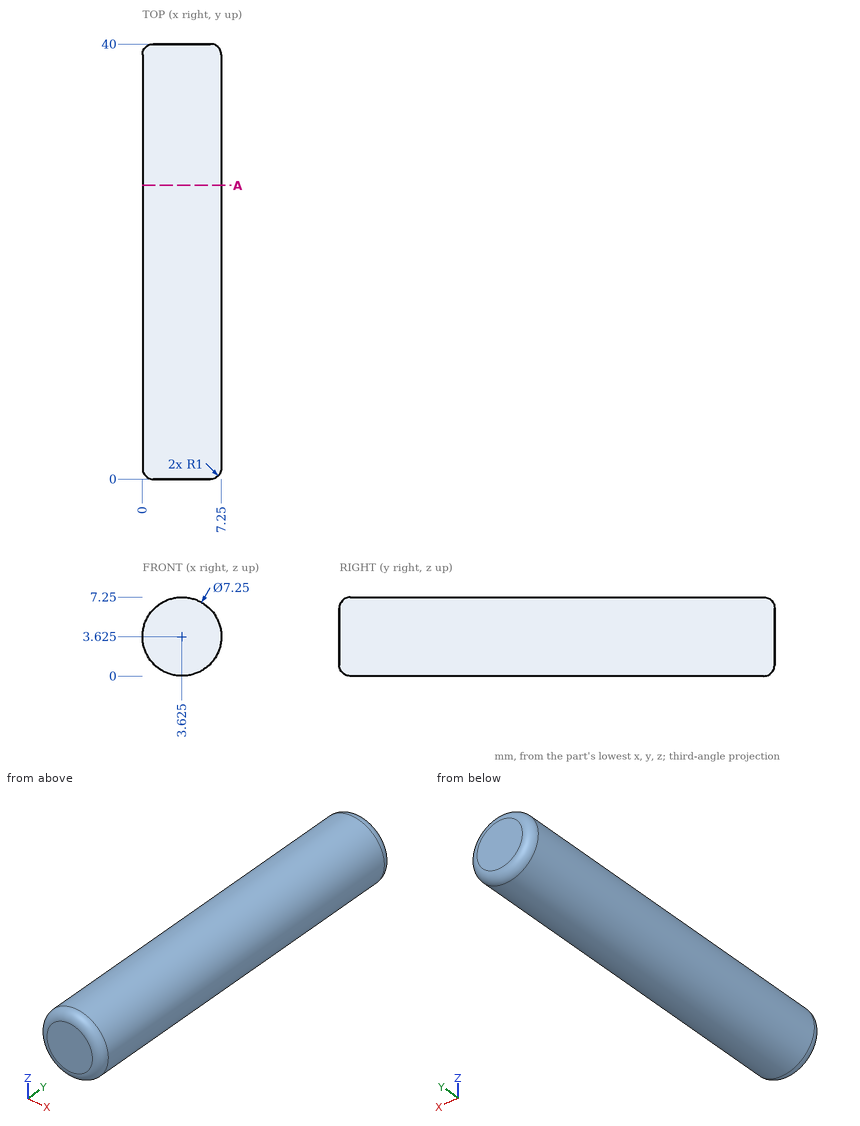
Design review of the part shown in the three views and the two pictorial views. Dimensions are in mm from the part's minimum x, y and z. Round coordinates to 2 decimals unless told otherwise and drop trailing zeros. Order: outer loops, then holes, each group sorted by start corner. A loop starts at its lowest first (then second) coordinate and runs counter-clockwise, first axis right, second up. Notation, with made-up numbers: (42.25, 7.25) - (57.25, 7.25) arc R22 cw to (57.25, 24.25) - close; hole circle Ø10 at (88.5, -19). An arc over 180 degrees is marked (long way). Answer in a Markdown table with one row per item.
(1) Clearance check with flat-ended pins moving along their axes: P1, Ø3, axis at x = 2, y = 5.5, coming from the -Z side; P2, Ø1.5, axis at x = 2.5, y = 34, coming from the +Z side. State where each tip first meets the part, or that it passes through.
Result set:
| item | result |
|---|---|
| P1 | stops at z = 0 |
| P2 | stops at z = 7.23 |
(2) Take a section at A-A on y = 27. Write out the cut boundary in (x, z) (3 decimals), plus the area to 3 significant figures.
Result set:
| item | result |
|---|---|
| outline | circle Ø7.25 at (3.625, 3.625) |
| area | 41.3 mm2 |
(3) For line 1 (Z direction, x = 3.5, y = 16); line 2 (Y direction, x = 5.5, z = 6.25); line 3 (X direction, y = 38, z = 5.5), list the stretches that pass through material, from the lowest coordinate up. Write a range as from..to.
Result set:
| item | result |
|---|---|
| line 1 | z = 0..7.25 |
| line 2 | y = 0.2..39.8 |
| line 3 | x = 0.52..6.73 |
